Print and shaded views of the part. All mm, measured from the part's lowest x, y and z. A direction names the side the tool comes from. Coordinates: 2 decimals unless noted, no trailing zeros. Order: outer loops, then holes, each group sorted by start corner. A loop starts at its lowest first (then second) coordinate and runs counter-clockwise, first axis right, second up. Notation, with made-up numbers: M -38,79.25 L 11,79.25 A17 ccw 11,94.25 Z; hole C 33.25,-22.75 d5. An arc over 180 degrees is marked long. Use a Markdown table: item, result. Add a question column.
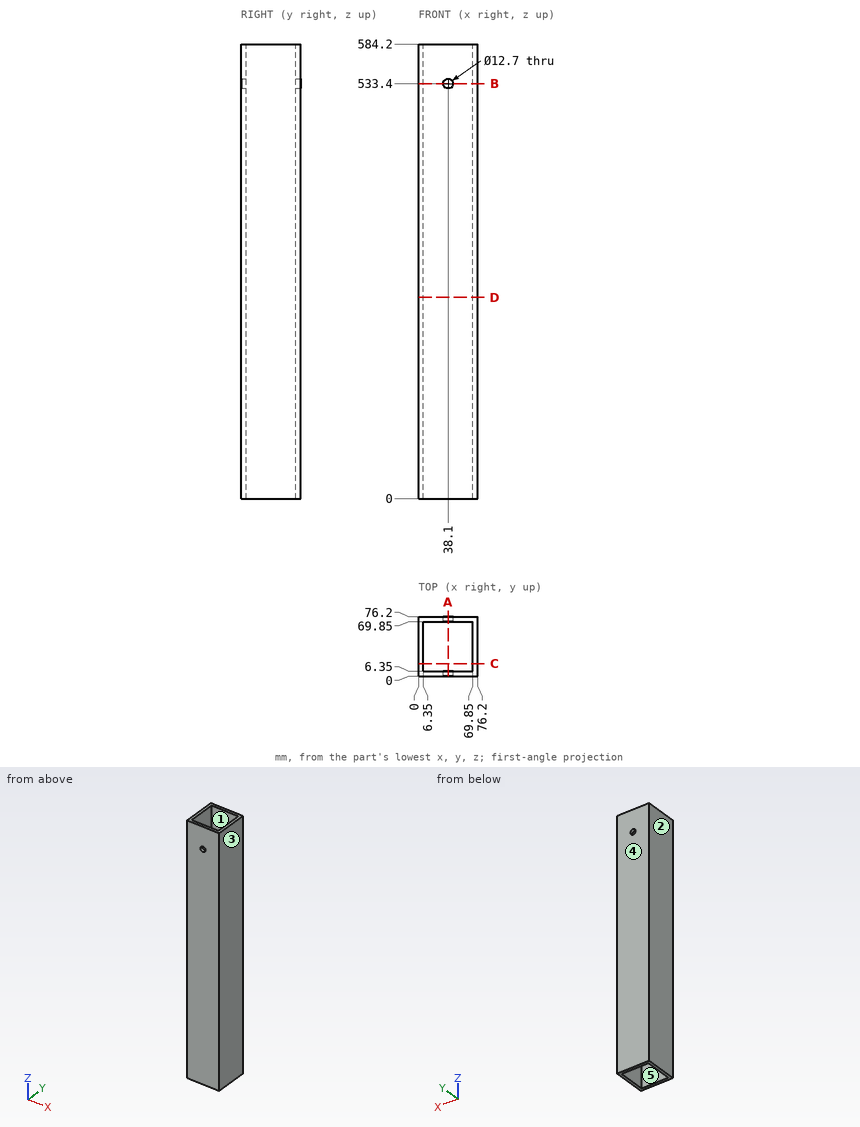
(1) Which spindle directions (+Z, -Z, +X, -X, +Y, -Y) get a long thin tool onto all of the face, cutting with end or side? Do the marked faces 1 and 2. Say none if no direction does.
(2) Mould opens along X. For the marked faces 3, 4 and 5 say: released by +X, released by -X, zero draft, split by the parting line, or undercut.
(3) Drill centre lines: line 1 along Y through (x, z) = (30.5, 118); line 2 along Z through (x, y) = (38.1, 4.75); line 3 along X through (y, z) = (4.75, 533.4). Where is each one in solid material? Low to high. Write a range as from..to.
(4) Slice it at A-A on x = 38.1. Give the cut face in (y, z).
(5) Slice it at D-D on z = 258.5. Give the cut face in (x, y), and give its area (3 significant figures).
(6) Slice it at B-B on z = 533.4. Give the cut face in (x, y).
(7) Slice it at C-C on y = 16. Give the cut face in (x, z), and give its area (3 significant figures).
Solutions:
| question | item | result |
|---|---|---|
| 1 | face 1 | +Z, -Z |
| 1 | face 2 | +Z, -Z, -X, +Y, -Y |
| 2 | face 3 | released by +X |
| 2 | face 4 | zero draft |
| 2 | face 5 | undercut |
| 3 | line 1 | 0..6.35, 69.85..76.2 |
| 3 | line 2 | 0..527.05, 539.75..584.2 |
| 3 | line 3 | 0..31.75, 44.45..76.2 |
| 4 | outline | M 0,0 L 6.35,0 L 6.35,527.05 L 0,527.05 Z; M 0,539.75 L 6.35,539.75 L 6.35,584.2 L 0,584.2 Z; M 69.85,0 L 76.2,0 L 76.2,527.05 L 69.85,527.05 Z; M 69.85,539.75 L 76.2,539.75 L 76.2,584.2 L 69.85,584.2 Z |
| 5 | outline | M 0,0 L 76.2,0 L 76.2,76.2 L 0,76.2 Z; hole M 6.35,6.35 L 69.85,6.35 L 69.85,69.85 L 6.35,69.85 Z |
| 5 | area | 1,770 mm² |
| 6 | outline | M 0,0 L 31.75,0 L 31.75,6.35 L 6.35,6.35 L 6.35,69.85 L 31.75,69.85 L 31.75,76.2 L 0,76.2 Z; M 44.45,0 L 76.2,0 L 76.2,76.2 L 44.45,76.2 L 44.45,69.85 L 69.85,69.85 L 69.85,6.35 L 44.45,6.35 Z |
| 7 | outline | M 0,0 L 6.35,0 L 6.35,584.2 L 0,584.2 Z; M 69.85,0 L 76.2,0 L 76.2,584.2 L 69.85,584.2 Z |
| 7 | area | 7,420 mm² |
